from build123d import *

# Parameters (mm, degrees)
PAD_DEPTH    = 8
THICKNESS_T  = -1.4
SKETCH001_R  = 8
POCKET_DEPTH = 5
FILLET001_R  = 0.5


with BuildPart() as part:
    # Sketch → Pad (new body)
    with BuildSketch(Plane.XY):
        with BuildLine():
            Line((-64.916876, -10), (4.583124, -10))
            ThreePointArc((4.583124, -10), (8.118658, -8.535534), (9.583124, -5))
            Line((9.583124, -5), (9.583124, 5))
            ThreePointArc((9.583124, 5), (8.118658, 8.535534), (4.583124, 10))
            Line((4.583124, 10), (-64.916876, 10))
            ThreePointArc((-73.208438, 12.5), (-69.247003, 10.638593), (-64.916876, 10))
            ThreePointArc((-73.208438, 12.5), (-96.5, 0), (-73.208438, -12.5))
            ThreePointArc((-64.916876, -10), (-69.247003, -10.638593), (-73.208438, -12.5))
        make_face()
    extrude(amount=PAD_DEPTH)

    # Thickness
    thickness_openings = [part.faces().sort_by_distance(p)[0] for p in [
        (-45.837274, 0, 8),
    ]]
    offset(amount=THICKNESS_T, openings=thickness_openings)

    # Sketch001 (on Face19 of Thickness) → Pocket (cut)
    with BuildSketch(Plane.XY.offset(1.4)):
        Circle(SKETCH001_R)
    extrude(amount=-POCKET_DEPTH, mode=Mode.SUBTRACT)

    # Fillet001
    fillet001_edges = [part.edges().sort_by_distance(p)[0] for p in [
        (-95.1, 0, 1.4),
    ]]
    fillet(fillet001_edges, radius=FILLET001_R)


solid = part.part
Geometry check sheet. Reference: the model listing, model coordinates, mm. A direction names the side the tool comes from. Give positions to 0.01 mm unless a question says otherwise; leave off trailing zeros. Write each loop counter-clockwise with the first axis right and the second up, starting at its lowest first coordinate (ties: lowest second). Pieces come first, ordered by that corner, then holes. Notation, with made-up numbers: (3, 47) - (44, 47) arc R29 cw to (44, 86) - close; hole circle Ø4 at (-3, 81). An arc over 180 degrees is marked (long way). Put each result on its own line as item: value.
1. Thickness scan on line 1 (Y direction, x = -29.5, z = 6.25); line 2 (Y direction, x = 0, z = 0.4); line 3 (Z direction, x = -62, y = 7). Record the ranges inside material, lowest first.
Ans:
line 1: y = -10 to -8.6, 8.6 to 10
line 2: y = -10 to -8, 8 to 10
line 3: z = 0 to 1.4
2. Set-up check for faces 5 (the flat face through (-48, -9, 8)), 6 (the flat face through (-30, 10, 4)), 7 (the flat face through (8.183, 0, 5)), 8 (the cylindrical face through (-1.73, -7.81, 0.71)), 9 (the flat face through (-31, -10, 4)): record each of +Z, -Z, +X, -X, +Y, -Y from which the full face is reachable in a straight line by a thin tool's end or side.
Ans:
face 5: +Z, +X, -X, +Y, -Y
face 6: +Z, -Z, +X, +Y
face 7: +Z
face 8: +Z, -Z
face 9: +Z, -Z, +X, -Y
3. Draft check along Y on faces 1 (the cylindrical face through (7.101, -7.573, 4.907)), 2 (the flat face through (-56, 0, 1.4)), 3 (the flat face through (9.583, 0, 4)), 4 (the cylindrical face through (8.157, 8.496, 3.944)). Enter one of: +Y half, -Y half, draft (parallel to the pull), parting line (faces both ways), or undercut.
Ans:
face 1: undercut
face 2: undercut
face 3: draft
face 4: +Y half
4. Sectioned sample at B-B, the plane z = 4.5. Enter the section's corners in (x, y), plus the area to 3 significant figures.
Ans:
outline: (-73.21, -12.5) arc R15 cw to (-64.92, -10) - (4.58, -10) arc R5 ccw to (9.58, -5) - (9.58, 5) arc R5 ccw to (4.58, 10) - (-64.92, 10) arc R15 cw to (-73.21, 12.5) arc R15 ccw (long way) to start; hole (-73.98, -11.33) arc R16.4 cw to (-64.92, -8.6) - (4.58, -8.6) arc R3.6 ccw to (8.18, -5) - (8.18, 5) arc R3.6 ccw to (4.58, 8.6) - (-64.92, 8.6) arc R16.4 cw to (-73.98, 11.33) arc R13.6 ccw (long way) to start
area: 340 mm²
5. Go/stop test with flat-tipped pins: pin 1 (1.5 mm diameter, centred on x = -28.5, z = 5.5, fed in from +Y); pin 2 (1.5 mm diameter, centred on x = -24.5, y = -4.5, fed in from +Z); pin 3 (9.5 mm diameter, centred on x = 0, y = 0, fed in from -Z); pin 4 (1 mm diameter, centred on y = -3, z = 1, fed in from -X). Record where each tip stops, or that it passes through.
Ans:
pin 1: stops at y = 10
pin 2: stops at z = 1.4
pin 3: passes through
pin 4: stops at x = -96.29
6. Sectioned sample at C-C, the plane x = -30. Enter the section's corners in (y, z), plus the area to 3 significant figures.
Ans:
outline: (-10, 0) - (10, 0) - (10, 8) - (8.6, 8) - (8.6, 1.9) arc R0.5 cw to (8.1, 1.4) - (-8.1, 1.4) arc R0.5 cw to (-8.6, 1.9) - (-8.6, 8) - (-10, 8) - close
area: 46.6 mm²
7. Sectioned sample at A-A, the plane x = 0. Enter the section's corners in (y, z).
Ans:
outline: (-10, 0) - (-8, 0) - (-8, 1.4) - (-8.1, 1.4) arc R0.5 cw to (-8.6, 1.9) - (-8.6, 8) - (-10, 8) - close; (8, 0) - (10, 0) - (10, 8) - (8.6, 8) - (8.6, 1.9) arc R0.5 cw to (8.1, 1.4) - (8, 1.4) - close
